Source: CAD feature listing. Evaluate the final solid. Frame: model axes, mm. Face numbers are marked on the shaded views. Round coordinates to 2 decimals unless told otherwise and drop trailing zeros. Loops run counter-clockwise (first coordinate to the right, second up) from the corner with the lowest first, then second, coordinate; pieces in that order, holes last.
Item 1: Section query C-C on z = -8.5. Return loops of the section in (x, y).
Item 2: Pull-direction query (X, two-part tool) for the marked faces 1, 2 and 3; classes: released by +X, released by -X, zero draft, split by the parting line, or undercut.
Item 3: Section query A-A on x = 0. Return loops of the section in (y, z).
Item 4: Ray query, L1, parallel to Z at x = 0, y = 13.5; L2, parallel to X at y = 14.5, z = -3.5; L3, parallel to Z at x = 12, y = 13. Return the intervals inside material, ascending.
Item 5: First-contact query: P1, Ø2, axis at y = 15.5, z = 26.5, coming from the +X side; P2, Ø8, axis at x = -46.5, y = 13, coming from the +Z side; P3, Ø1.5, axis at y = 12.5, z = -17.5, coming from the -X side. Flat tips, straight axial feed; report the tip coordinate or a pass-through.
Item 6: Section query D-D on x = 35.5. Return loops of the section in (y, z), then the cut area to 3 significant figures.
Item 7: Section query B-B on y = 7. Return loops of the section in (x, z), then the cut area to 3 significant figures.
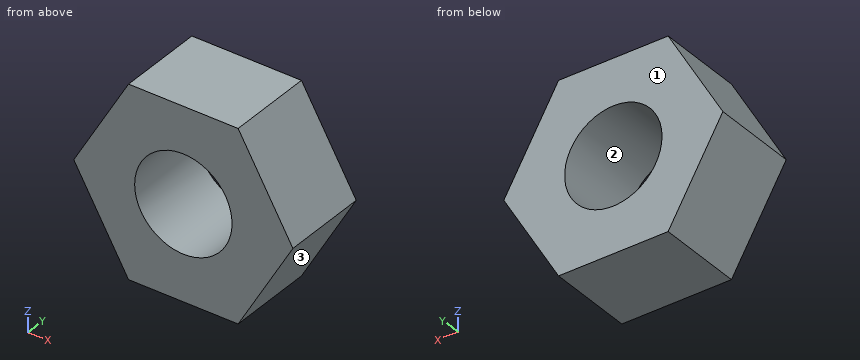
```python
from build123d import *

# Parameters (mm, degrees)
F1_DEPTH = 46.99
F2_R     = 26.387041
F3_DEPTH = 46.991


with BuildPart() as f1:
    # F0 (on Front) → F1 (new body)
    with BuildSketch(Plane.XZ):
        Polygon((-29.690725, -51.425844), (29.690725, -51.425844), (59.38145, 0), (29.690725, 51.425844), (-29.690725, 51.425844), (-59.38145, 0), align=None)
    extrude(amount=-F1_DEPTH)

    # F2 (on face) → F3 (cut, through all)
    with BuildSketch(Plane(origin=(0, 46.99, 0), x_dir=(-1, 0, 0), z_dir=(0, 1, 0))):
        Circle(F2_R)
    extrude(amount=-F3_DEPTH, mode=Mode.SUBTRACT)


solid = f1.part
```
Data:
1. outline: (-54.47, 0) - (-24.98, 0) - (-24.98, 46.99) - (-54.47, 46.99) - close; (24.98, 0) - (54.47, 0) - (54.47, 46.99) - (24.98, 46.99) - close
2. face 1: zero draft
2. face 2: undercut
2. face 3: released by +X
3. outline: (0, -51.43) - (46.99, -51.43) - (46.99, -26.39) - (0, -26.39) - close; (0, 26.39) - (46.99, 26.39) - (46.99, 51.43) - (0, 51.43) - close
4. L1: z = -51.43 to -26.39, 26.39 to 51.43
4. L2: x = -57.36 to -26.15, 26.15 to 57.36
4. L3: z = -51.43 to -23.5, 23.5 to 51.43
5. P1: stops at x = 44.66
5. P2: stops at z = 29.24
5. P3: stops at x = -49.71
6. outline: (0, -41.36) - (46.99, -41.36) - (46.99, 41.36) - (0, 41.36) - close
6. area: 3,890 mm2
7. outline: (-59.38, 0) - (-29.69, -51.43) - (29.69, -51.43) - (59.38, 0) - (29.69, 51.43) - (-29.69, 51.43) - close; hole circle Ø52.77 at (0, 0)
7. area: 6,970 mm2
